Read the model definition and answer for the solid it produces. Units are mm, in the model's axes. Round coordinates to 2 decimals unless told otherwise and drop trailing zeros. Loops run counter-clockwise (first coordinate to the right, second up) from the corner with the lowest first, then second, coordinate; pieces in that order, holes last. Notation, with made-up numbers: (46.5, -4) -> (52.5, -4) arc R5 cw to (52.5, 3) -> close; hole circle Ø4 at (20.25, 25). An arc over 180 degrees is marked (long way). Put each result on its own line as item: value.
Autodesk Inventor part; units mm, degrees
ref_plane "YZ Plane" through (0, 0, 0) normal (1, 0, 0) x (0, 1, 0)
ref_plane "XZ Plane" through (0, 0, 0) normal (0, 1, 0) x (-1, 0, 0)
ref_plane "XY Plane" through (0, 0, 0) normal (0, 0, 1) x (1, 0, 0)
sketch "Sketch1" plane through (0, 0, 0) normal (0, 0, 1) x (1, 0, 0)
  circle A0 centre (0, 0) radius 2
  dimension "Diameter" = 4
extrude "Extrusion1" add sketch "Sketch1" along normal blind 62.52
sketch "Sketch2" plane through (0, 0, 62.52) normal (0, 0, 1) x (1, 0, 0)
  circle A0 centre (0, 0) radius 2
extrude "Extrusion2" add sketch "Sketch2" along normal blind 2.48 draft 45
sketch "Sketch3" plane through (0, 0, 65) normal (0, 0, 1) x (1, 0, 0)
  circle A0 centre (0, 0) radius 4.48
  circle A1 centre (0, 0) radius 1.4434 construction
  line L0 (0.6042, 1.3108) -> (1.4373, 0.1322)
  line L1 (1.4373, 0.1322) -> (0.8331, -1.1787)
  line L2 (0.8331, -1.1787) -> (-0.6042, -1.3108)
  line L3 (-0.6042, -1.3108) -> (-1.4373, -0.1322)
  line L4 (-1.4373, -0.1322) -> (-0.8331, 1.1787)
  line L5 (-0.8331, 1.1787) -> (0.6042, 1.3108)
  dimension "Hex_Width" = 2.5
extrude "Extrusion3" cut sketch "Sketch3" against normal blind 1.5 contours L0 L1 L2 L3 L4 L5
chamfer "Chamfer2" distance 0.4 angle 45 1 edges at (-2, 0, 0)
fillet "Fillet1" radius 0.1 1 edges at (-4.48, 0, 65)
thread "Thread2"
equation "\"d13\" = Chamfer"
equation "\"Thread_Length\" = 7.52"
properties part number "SCREW, FLAT HD, P, 12_9, M4X0_7X65MM" material "Steel"
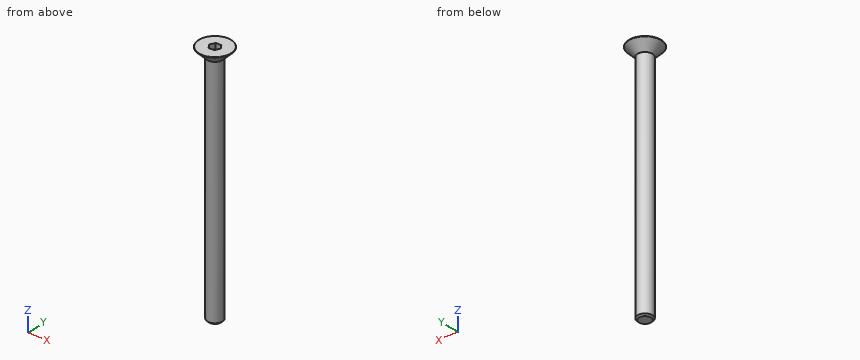
Item 1: Flat-ended cylindrical pins translate along their axes: pin 1 Ø1.5 at (y, z) = (0, 39) entering from -X; pin 2 Ø1 at (x, y) = (-1, 3.5) entering from -Z; pin 3 Ø3 at (y, z) = (3, 7) entering from +X. Find the tip coordinate at first contact, or state that the pin passes through.
Derived:
pin 1: stops at x = -2
pin 2: stops at z = 63.66
pin 3: stops at x = 1.32
Item 2: Find the intervals of material crossed by line 1 along X through (y, z) = (1.5, 18); line 2 along Z through (x, y) = (-0.5, 0.75), in increasing order.
Derived:
line 1: x = -1.32 to 1.32
line 2: z = 0 to 63.5
Item 3: The part is cut by section B-B (z = 55). Determine the outline of the cut face in (x, y), then the cut area to 3 significant figures.
Derived:
outline: circle Ø4 at (0, 0)
area: 12.6 mm^2
Item 4: The part is cut by section A-A (x = 0). Determine the outline of the cut face in (y, z), then the cut area to 3 significant figures.
Derived:
outline: (-4.31, 64.83) -> (-2, 62.52) -> (-2, 0.4) -> (-1.6, 0) -> (1.6, 0) -> (2, 0.4) -> (2, 62.52) -> (4.31, 64.83) arc R0.1 ccw to (4.24, 65) -> (1.26, 65) -> (1.26, 63.5) -> (-1.26, 63.5) -> (-1.26, 65) -> (-4.24, 65) arc R0.1 ccw to start
area: 262 mm^2
